Work out the finished part from the listing and answer in its coordinate system (mm). Face numbers are marked on the shaded views. Round coordinates to 2 decimals unless told otherwise and drop trailing zeros. Order: outer loops, then holes, each group sorted by start corner. A loop starts at its lowest first (then second) coordinate and runs counter-clockwise, first axis right, second up. Notation, with made-up numbers: (19, -9) - (27, -9) arc R16 cw to (27, 20) - close; hole circle Ø1 at (57.5, 10.5). An arc over 180 degrees is marked (long way). Put each result on its own line as item: value.
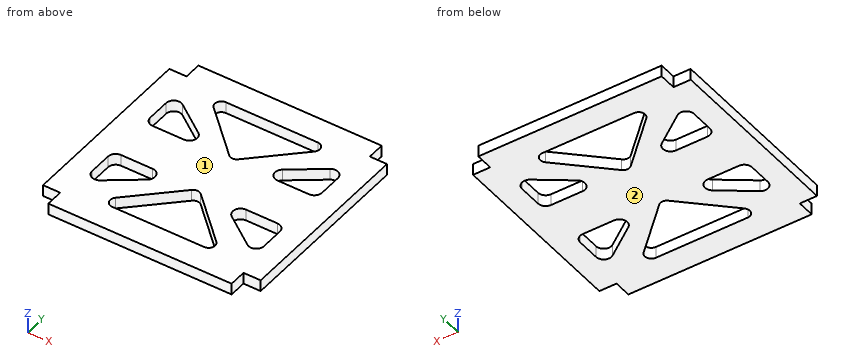
```python
from build123d import *

# Parameters (mm, degrees)
F1_DEPTH = 5
F2_R     = 2.839641
F3_R     = 3.37981


with BuildPart() as f1:
    # F0 (on Top) → F1 (new body)
    with BuildSketch(Plane.XY):
        Polygon((-40, -47.5), (40, -47.5), (40, -40), (47.5, -40), (47.5, 40), (40, 40), (40, 47.5), (-40, 47.5), (-40, 40), (-47.5, 40), (-47.5, -40), (-40, -40), align=None)
        Polygon((-37.5, -30), (-37.5, -10), (-10, -10), align=None, mode=Mode.SUBTRACT)
        Polygon((0, -10), (27.139446, -35.976308), (-27.139446, -35.976308), align=None, mode=Mode.SUBTRACT)
        Polygon((37.5, -30), (10, -10), (37.5, -10), align=None, mode=Mode.SUBTRACT)
        Polygon((-10, 10), (-37.5, 10), (-37.5, 30), align=None, mode=Mode.SUBTRACT)
        Polygon((0, 10), (-27.139446, 35.976308), (27.139446, 35.976308), align=None, mode=Mode.SUBTRACT)
        Polygon((37.5, 10), (10, 10), (37.5, 30), align=None, mode=Mode.SUBTRACT)
    extrude(amount=F1_DEPTH)

    # F2
    f2_edges = [f1.edges().sort_by_distance(p)[0] for p in [
        (27.139446, 35.976308, 2.5),
        (-27.139446, 35.976308, 2.5),
        (0, 10, 2.5),
        (0, -10, 2.5),
        (-27.139446, -35.976308, 2.5),
        (27.139446, -35.976308, 2.5),
    ]]
    fillet(f2_edges, radius=F2_R)

    # F3
    f3_edges = [f1.edges().sort_by_distance(p)[0] for p in [
        (37.5, 30, 2.5),
        (37.5, 10, 2.5),
        (10, -10, 2.5),
        (-37.5, -10, 2.5),
        (-10, -10, 2.5),
        (37.5, -10, 2.5),
        (-37.5, 30, 2.5),
        (37.5, -30, 2.5),
        (-10, 10, 2.5),
        (-37.5, 10, 2.5),
        (-37.5, -30, 2.5),
        (10, 10, 2.5),
    ]]
    fillet(f3_edges, radius=F3_R)


solid = f1.part
```
1) Straight lines are drawn through the part: L1, parallel to Y at x = 30.5, z = 3; L2, parallel to Y at x = -6, z = 2.9; L3, parallel to X at y = -25, z = 4.2 (3 decimals). For each, find the intervals that lie inside material, in ascending order. Write a range as from..to.
Findings below:
L1: y = -47.5..-24.91, -10..10, 24.91..47.5
L2: y = -47.5..-35.98, -15.74..15.74, 35.98..47.5
L3: x = -47.5..-37.077, -30.625..-15.672, 15.672..30.625, 37.077..47.5
2) A cutting plane is placed at D-D on z = 2.4. Give the number of separate pieces and of enclosed holes in the cut face, then the cut area to 3 significant figures.
Findings below:
separate pieces: 1
enclosed holes: 6
area: 6,470 mm2
3) Given pin 1 Ø2.5 at (y, z) = (-44.5, 1.5) entering from -X; pin 2 Ø2.5 at (y, z) = (-44, 2.5) entering from +X; pin 3 Ø1.5 at (x, z) = (43.5, 1.5) entering from -Y, each flat-ended and moving along its own axis, determine where each tip first touches the part or whether it passes through.
Findings below:
pin 1: stops at x = -40
pin 2: stops at x = 40
pin 3: stops at y = -40
4) A cutting plane is placed at A-A on y = -21. Write down the section's boundary in (x, z) (3 decimals).
Findings below:
outline: (-47.5, 0) - (-37.5, 0) - (-37.5, 5) - (-47.5, 5) - close; (-25.125, 0) - (-11.493, 0) - (-11.493, 5) - (-25.125, 5) - close; (11.493, 0) - (25.125, 0) - (25.125, 5) - (11.493, 5) - close; (37.5, 0) - (47.5, 0) - (47.5, 5) - (37.5, 5) - close
5) A cutting plane is placed at B-B on x = -28. Write down the section's boundary in (y, z).
Findings below:
outline: (-47.5, 0) - (-23.09, 0) - (-23.09, 5) - (-47.5, 5) - close; (-10, 0) - (10, 0) - (10, 5) - (-10, 5) - close; (23.09, 0) - (47.5, 0) - (47.5, 5) - (23.09, 5) - close
6) For a pull along Z with two mould halves and no side action, classify the marked faces 1 and 2 as pulls with the +Z half, pulls with the -Z half, needs draft (parallel to the pull), parting line crosses it, or undercut.
Findings below:
face 1: pulls with the +Z half
face 2: pulls with the -Z half
7) A cutting plane is placed at C-C on y = -33.5. Write down the section's boundary in (x, z).
Findings below:
outline: (-47.5, 0) - (-22.88, 0) - (-22.88, 5) - (-47.5, 5) - close; (22.88, 0) - (47.5, 0) - (47.5, 5) - (22.88, 5) - close
